from build123d import *

# Parameters (mm, degrees)
SKETCH1_W             = 23.2
SKETCH1_H             = 41.57
BOSS_EXTRUDE1_DEPTH   = 1.5
SKETCH2_W             = 23.2
SKETCH2_H             = 3
BOSS_EXTRUDE2_DEPTH   = 4
SKETCH3_W             = 23.2
SKETCH3_H             = 3
CUT_EXTRUDE1_DEPTH    = 1.2
SKETCH4_W             = 23.2
SKETCH4_H             = 3
CUT_EXTRUDE2_DEPTH    = 1.2
SKETCH5_R             = 1.5
CUT_EXTRUDE3_DEPTH    = 48.773474858
SKETCH7_W             = 23.2
SKETCH7_H             = 5.7
CUT_EXTRUDE4_DEPTH    = 48.922384123
SKETCH8_W             = 15.2
SKETCH8_H             = 4
CUT_EXTRUDE5_DEPTH    = 44.071416276
SKETCH9_W             = 6.6
SKETCH9_H             = 5.7
CUT_EXTRUDE6_DEPTH    = 48.773474858
FILLET1_R             = 2
BODY_MOVE_COPY1_ANGLE = 90


with BuildPart() as part:
    # Sketch1 → Boss-Extrude1 (new body)
    with BuildSketch(Plane(origin=(0, 0, 0), x_dir=(1, 0, 0), z_dir=(0, 1, 0))):
        with Locations((11.6, 20.785)):
            Rectangle(SKETCH1_W, SKETCH1_H)
    extrude(amount=BOSS_EXTRUDE1_DEPTH)

    # Sketch2 → Boss-Extrude2 (add)
    with BuildSketch(Plane(origin=(0, 1.5, 0), x_dir=(1, 0, 0), z_dir=(0, 1, 0))):
        with Locations((11.6, 34.37)):
            Rectangle(SKETCH2_W, SKETCH2_H)
        with Locations((11.6, 7.2)):
            Rectangle(SKETCH2_W, SKETCH2_H)
    extrude(amount=BOSS_EXTRUDE2_DEPTH)

    # Sketch3 → Cut-Extrude1 (cut)
    with BuildSketch(Plane.XY.offset(-32.87)):
        with Locations((11.6, 3)):
            Rectangle(SKETCH3_W, SKETCH3_H)
    extrude(amount=-CUT_EXTRUDE1_DEPTH, mode=Mode.SUBTRACT)

    # Sketch4 → Cut-Extrude2 (cut)
    with BuildSketch(Plane(origin=(0, 0, -8.7), x_dir=(-1, 0, 0), z_dir=(0, 0, -1))):
        with Locations((-11.6, 3)):
            Rectangle(SKETCH4_W, SKETCH4_H)
    extrude(amount=-CUT_EXTRUDE2_DEPTH, mode=Mode.SUBTRACT)

    # Sketch5 → Cut-Extrude3 (cut, through all)
    with BuildSketch(Plane(origin=(0, 1.5, 0), x_dir=(1, 0, 0), z_dir=(0, 1, 0))):
        with Locations(Location((11.6, 38.72, 0), (0, 0, 270))):
            Circle(SKETCH5_R)
        with Locations(Location((11.6, 2.85, 0), (0, 0, 270))):
            Circle(SKETCH5_R)
    extrude(amount=-CUT_EXTRUDE3_DEPTH, mode=Mode.SUBTRACT)

    # Sketch7 → Cut-Extrude4 (cut, through all)
    with BuildSketch(Plane(origin=(0, 0, 0), x_dir=(1, 0, 0), z_dir=(0, 1, 0))):
        with Locations((11.6, 2.85)):
            Rectangle(SKETCH7_W, SKETCH7_H)
    extrude(amount=CUT_EXTRUDE4_DEPTH, mode=Mode.SUBTRACT)

    # Sketch8 → Cut-Extrude5 (cut, through all)
    with BuildSketch(Plane.XY.offset(-5.7)):
        with Locations((11.6, 3.5)):
            Rectangle(SKETCH8_W, SKETCH8_H)
    extrude(amount=-CUT_EXTRUDE5_DEPTH, mode=Mode.SUBTRACT)

    # Sketch9 → Cut-Extrude6 (cut, through all)
    with BuildSketch(Plane(origin=(0, 1.5, 0), x_dir=(1, 0, 0), z_dir=(0, 1, 0))):
        with Locations((3.3, 38.72)):
            Rectangle(SKETCH9_W, SKETCH9_H)
        with Locations((19.9, 38.72)):
            Rectangle(SKETCH9_W, SKETCH9_H)
    extrude(amount=-CUT_EXTRUDE6_DEPTH, mode=Mode.SUBTRACT)

    # Fillet1
    fillet1_edges = [part.edges().sort_by_distance(p)[0] for p in [
        (6.6, 0.75, -41.57),
        (6.6, 0.75, -35.87),
        (16.6, 0.75, -41.57),
        (16.6, 0.75, -35.87),
    ]]
    fillet(fillet1_edges, radius=FILLET1_R)


with BuildPart() as part_1:
    # Body-Move/Copy1: moved
    add(part.part.rotate(Axis((0, 2.75, -20.7), (1, 0, 0)), BODY_MOVE_COPY1_ANGLE))


solid = part_1.part
Design review of the part built by this model. Coordinates are the model's own, in mm. A direction names the side the tool comes from. Give positions to 0.01 mm unless a question says otherwise; leave off trailing zeros. Order: outer loops, then holes, each group sorted by start corner. A loop starts at its lowest first (then second) coordinate and runs counter-clockwise, first axis right, second up.
1. Add section A-A, the plane z = -20.1. State the section outline as (x, y) points, then the cut area to 3 significant figures.
Solution:
outline: (0, -12.25) - (4, -12.25) - (4, -10.45) - (0, -10.45) - close; (0, 16.12) - (4, 16.12) - (4, 17.92) - (0, 17.92) - close; (19.2, -12.25) - (23.2, -12.25) - (23.2, -10.45) - (19.2, -10.45) - close; (19.2, 16.12) - (23.2, 16.12) - (23.2, 17.92) - (19.2, 17.92) - close
area: 28.8 mm2
2. To check wall thickness, follow L1, parallel to X at y = 20.77, z = -22.5; L2, parallel to Z at x = 19.75, y = 16; L3, parallel to Z at x = 12.75, y = 12. State the ranges of each line that lie inside material, in increasing order.
Solution:
L1: x = 6.6 to 10.1, 13.1 to 16.6
L2: z = -23.45 to -21.95, -18.95 to -17.95
L3: z = -23.45 to -21.95
3. Tool access review of faces 4 (the flat face through (6.6, 21, -23)), 5 (the flat face through (2, 15.5, -18.95)), 6 (the flat face through (4, -11, -20)), 7 (the flat face through (21.2, -9.25, -18.5)): name each direction out of +Z, -Z, +X, -X, +Y, -Y from which nothing blocks a thin tool from reaching the whole face with its end or side.
Solution:
face 4: +Z, -Z, -X, +Y
face 5: +X, -X
face 6: +Z, +Y, -Y
face 7: +Z, +X, -X
4. Add section C-C, the plane x = 11.6. State the section outline as (y, z) points.
Solution:
outline: (-12.25, -23.45) - (19.27, -23.45) - (19.27, -21.95) - (-12.25, -21.95) - close; (22.27, -23.45) - (23.62, -23.45) - (23.62, -21.95) - (22.27, -21.95) - close
5. Add section D-D, the plane y = -10. State the section outline as (x, z) points, then the cut area to 3 significant figures.
Solution:
outline: (0, -23.45) - (23.2, -23.45) - (23.2, -21.95) - (0, -21.95) - close; (0, -18.95) - (4, -18.95) - (4, -17.95) - (0, -17.95) - close; (19.2, -18.95) - (23.2, -18.95) - (23.2, -17.95) - (19.2, -17.95) - close
area: 42.8 mm2
6. Add section B-B, the plane y = 20.77. State the section outline as (x, z) points, then the cut area to 3 significant figures.
Solution:
outline: (6.6, -23.45) - (10.1, -23.45) - (10.1, -21.95) - (6.6, -21.95) - close; (13.1, -23.45) - (16.6, -23.45) - (16.6, -21.95) - (13.1, -21.95) - close
area: 10.5 mm2
7. For pin 1 Ø8 at (x, y) = (9.5, -6.5) entering from +Z; pin 2 Ø2.5 at (x, z) = (20.5, -21.5) entering from +Y; pin 3 Ø0.8 at (y, z) = (21, -23) entering from +X, all flat-tipped, find the tip position at first contact; note any pin that passes through.
Solution:
pin 1: stops at z = -21.95
pin 2: stops at y = 17.92
pin 3: stops at x = 16.6
8. Mouldability with a two-part tool opening along X and no side actions: class faces 1 (the flat face through (2, 14.92, -18.5)), 2 (the flat face through (16.6, 21, -23)), 3 (the flat face through (4, 17, -20)) as +X half, -X half, draft (parallel to the pull), parting line (faces both ways), or undercut.
Solution:
face 1: draft
face 2: +X half
face 3: undercut
